Design review of the part built by this model. Coordinates are the model's own, in mm. A direction names the side the tool comes from. Give positions to 0.01 mm unless a question says otherwise; leave off trailing zeros. Write each loop counter-clockwise with the first axis right and the second up, starting at its lowest first coordinate (ties: lowest second). Pieces come first, ordered by that corner, then holes. Notation, with made-up numbers: M 80.25,14.5 L 118.25,14.5 A23 cw 118.25,51.5 Z; hole C -19.75,36 d7. An arc over 180 degrees is marked long. Answer in a Markdown table with one row per item.
```python
from build123d import *

# Parameters (mm, degrees)
SKETCH2_R   = 3.175
SKETCH2_R_2 = 2.4638


with BuildPart() as part:
    # Sweep-Thin1: sweep along a path in Sketch1
    with BuildLine(Plane(origin=(0, 0, 0), x_dir=(1, 0, 0), z_dir=(0, 1, 0))) as sweep_thin1_path:
        Line((-257.7, 36), (-16, 36))
        ThreePointArc((-16, 36), (-4.686291501, 31.313708499), (0, 20))
        Line((0, 20), (0, 0))
    # Sketch2 → Sweep-Thin1 (sweep)
    with BuildSketch(Plane.XY):
        Circle(SKETCH2_R)
        Circle(SKETCH2_R_2, mode=Mode.SUBTRACT)
    sweep(path=sweep_thin1_path.line)


solid = part.part
```
1) Add section C-C (z = -3). Write out the cut boundary in (x, y) (3 decimals), and give its area (3 significant figures).
Geometry says:
| item | result |
|---|---|
| outline | C 0,0 d6.35; hole C 0,0 d4.928 |
| area | 12.6 mm^2 |
2) For faces 1 (the face through (-135.16, 0.95, -39.03)), 2 (the face through (-2.46, 0.11, -9.86)), list the 3-axis set-ups (+Z, -Z, +X, -X, +Y, -Y) from which the entire face can be reached by the end or side of a thin tool; tool diameter is ignored.
Geometry says:
| item | result |
|---|---|
| face 1 | -X |
| face 2 | +Z |
3) Add section B-B (x = -34). Write out the cut boundary in (y, z) (3 decimals), and give its area (3 significant figures).
Geometry says:
| item | result |
|---|---|
| outline | C 0,-36 d6.35; hole C 0,-36 d4.928 |
| area | 12.6 mm^2 |
4) The part is to be moulded in two halves that separate along Z. For faces 3 (the face through (-135.16, 0.74, -38.35)), 4 (the face through (2, -2, 0)), 5 (the face through (-257.7, 2, -34)), say which applies: released by +Z, released by -Z, zero draft, split by the parting line, or undercut.
Geometry says:
| item | result |
|---|---|
| face 3 | undercut |
| face 4 | released by +Z |
| face 5 | zero draft |
5) To check wall thickness, follow probe 1 along X at (y, z) = (0, -14) (3 decimals); probe 2 along Y at (x, z) = (-117, -36.5). State the ranges of each line that lie inside material, in increasing order. Write a range as [from, to].
Geometry says:
| item | result |
|---|---|
| probe 1 | [-3.175, -2.464], [2.464, 3.175] |
| probe 2 | [-3.14, -2.41], [2.41, 3.14] |
6) Insertion check: P1, Ø1, axis at y = -1.5, z = -16, coming from the +X side; P2, Ø2, axis at y = -1, z = -14.5, coming from the -X side (3 decimals); P3, Ø10, axis at x = -146, z = -28.5, coming from the +Y side. Each pin has a flat end and moves straight along its axis. Give the tip position at first contact, or say it passes through.
Geometry says:
| item | result |
|---|---|
| P1 | x = 3.01 |
| P2 | x = -3.175 |
| P3 | y = 1.96 |
7) Add section A-A (y = 0). Write out the cut boundary in (x, z) (3 decimals), and give its area (3 significant figures).
Geometry says:
| item | result |
|---|---|
| outline | M -257.7,-39.175 L -16,-39.175 A19.175 ccw 3.175,-20 L 3.175,0 L 2.464,0 L 2.464,-20 A18.464 cw -16,-38.464 L -257.7,-38.464 Z; M -257.7,-33.536 L -16,-33.536 A13.536 ccw -2.464,-20 L -2.464,0 L -3.175,0 L -3.175,-20 A12.825 cw -16,-32.825 L -257.7,-32.825 Z |
| area | 408 mm^2 |
